Geometry check sheet. Reference: the model listing, model coordinates, mm. Face numbers are marked on the shaded views. Coordinates: 2 decimals unless noted, no trailing zeros. Order: outer loops, then holes, each group sorted by start corner. A loop starts at its lowest first (then second) coordinate and runs counter-clockwise, first axis right, second up.
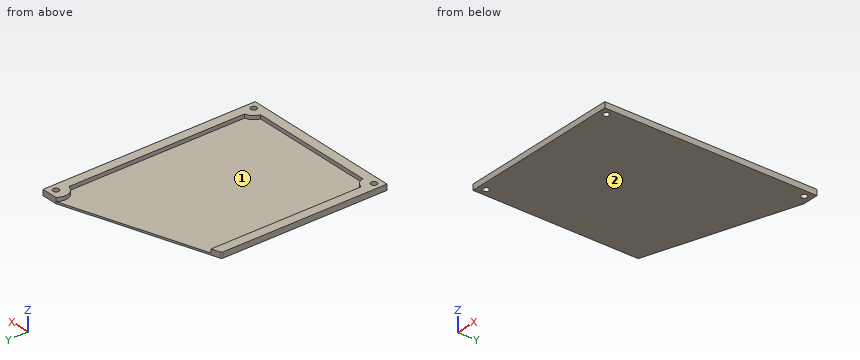
```python
from build123d import *

# Parameters (mm, degrees)
SKETCH_W           = 86.36
SKETCH_H           = 113.03
PAD_DEPTH          = 10
SKETCH001_R        = 1.6
POCKET_DEPTH       = 1
POCKET001_DEPTH    = 9
POCKET002_DEPTH    = 10.001
FILLET_R           = 1
FILLET_FACE20_R    = 1.6
POCKET003_DEPTH    = 9.001
POCKET003_FACE20_R = 1.6
POCKET004_DEPTH    = 9.001
POCKET004_FACE21_R = 1.6
POCKET005_DEPTH    = 9.001
POCKET005_FACE11_R = 1.6
POCKET006_DEPTH    = 7


with BuildPart() as part:
    # Sketch → Pad (new body)
    with BuildSketch(Plane.XY):
        Rectangle(SKETCH_W, SKETCH_H)
    extrude(amount=PAD_DEPTH)

    # Sketch001 (on Face6 of Pad) → Pocket (cut)
    with BuildSketch(Plane.XY.offset(10)):
        with Locations((-39.37, -52.705)):
            Circle(SKETCH001_R)
        with Locations((39.37, -52.705)):
            Circle(SKETCH001_R)
        with Locations((39.37, 52.705)):
            Circle(SKETCH001_R)
    extrude(amount=-POCKET_DEPTH, mode=Mode.SUBTRACT)

    # Sketch002 (on Face5 of Pocket) → Pocket001 (cut)
    with BuildSketch(Plane.XY.offset(10)):
        with BuildLine():
            Line((-38.18, 56.515), (34.734927, 56.515))
            ThreePointArc((34.734927, 56.515), (33.716611, 50.695226), (38.18, 46.824192))
            Line((38.18, -46.824192), (38.18, 46.824192))
            ThreePointArc((38.18, -46.824192), (35.127359, -48.462359), (33.489192, -51.515))
            Line((-33.489192, -51.515), (33.489192, -51.515))
            ThreePointArc((-33.489192, -51.515), (-35.127359, -48.462359), (-38.18, -46.824192))
            Line((-38.18, -46.824192), (-38.18, 56.515))
        make_face()
    extrude(amount=-POCKET001_DEPTH, mode=Mode.SUBTRACT)

    # Sketch003 (on Face2 of Pocket001) → Pocket002 (cut, through all)
    with BuildSketch(Plane(origin=(0, 0, 0), x_dir=(1, 0, 0), z_dir=(0, 0, -1))):
        Polygon((34.734927, -56.515), (-43.18, -31.515), (-75.693622, -36.778853), (-62.654191, -136.900963), (71.529642, -145.781613), align=None)
    extrude(amount=-POCKET002_DEPTH, mode=Mode.SUBTRACT)

    # Fillet
    fillet_edges = [part.edges().sort_by_distance(p)[0] for p in [
        (-43.18, 31.515, 5),
    ]]
    fillet(fillet_edges, radius=FILLET_R)

    # Fillet Face20 → Pocket003 (cut, through all)
    with BuildSketch(Plane(origin=(39.37, 52.705, 9), x_dir=(0, 1, 0), z_dir=(0, 0, 1))):
        Circle(FILLET_FACE20_R)
    extrude(amount=-POCKET003_DEPTH, mode=Mode.SUBTRACT)

    # Pocket003 Face20 → Pocket004 (cut, through all)
    with BuildSketch(Plane(origin=(39.37, -52.705, 9), x_dir=(0, 1, 0), z_dir=(0, 0, 1))):
        Circle(POCKET003_FACE20_R)
    extrude(amount=-POCKET004_DEPTH, mode=Mode.SUBTRACT)

    # Pocket004 Face21 → Pocket005 (cut, through all)
    with BuildSketch(Plane(origin=(-39.37, -52.705, 9), x_dir=(0, 1, 0), z_dir=(0, 0, 1))):
        Circle(POCKET004_FACE21_R)
    extrude(amount=-POCKET005_DEPTH, mode=Mode.SUBTRACT)

    # Pocket005 Face11 → Pocket006 (cut)
    with BuildSketch(Plane(origin=(4.164338, -17.509982, 10), x_dir=(0, 1, 0), z_dir=(0, 0, 1))):
        with BuildLine():
            Line((50.629296, 42.344338), (49.247815, 46.649859))
            ThreePointArc((49.247815, 46.649859), (48.8849, 47.152274), (48.295629, 47.344338))
            Line((48.295629, 47.344338), (-39.005018, 47.344338))
            Line((-39.005018, 47.344338), (-39.005018, -39.015662))
            Line((-39.005018, -39.015662), (74.024982, -39.015662))
            Line((74.024982, -39.015662), (74.024982, -30.570589))
            ThreePointArc((74.024982, -30.570589), (68.205208, -29.552273), (64.334174, -34.015662))
            Line((64.334174, -34.015662), (-29.31421, -34.015662))
            ThreePointArc((-29.31421, -34.015662), (-30.952377, -30.963021), (-34.005018, -29.324854))
            Line((-34.005018, -29.324854), (-34.005018, 37.65353))
            ThreePointArc((-34.005018, 37.65353), (-30.952377, 39.291697), (-29.31421, 42.344338))
            Line((-29.31421, 42.344338), (50.629296, 42.344338))
        make_face()
        with Locations((-35.195018, -35.205662)):
            Circle(POCKET005_FACE11_R, mode=Mode.SUBTRACT)
        with Locations((70.214982, -35.205662)):
            Circle(POCKET005_FACE11_R, mode=Mode.SUBTRACT)
        with Locations((-35.195018, 43.534338)):
            Circle(POCKET005_FACE11_R, mode=Mode.SUBTRACT)
    extrude(amount=-POCKET006_DEPTH, mode=Mode.SUBTRACT)


solid = part.part
```
Item 1: Sectioned sample at C-C (y = -41). Record the cut outline in (x, z).
Item 2: Depth check by flat-ended pin: P1, Ø1.6, axis at x = -4, z = 1.5, coming from the +Y side; P2, Ø1, axis at x = 20.5, y = 9.5, coming from the +Z side; P3, Ø1.5, axis at x = -3, z = 0.5, coming from the +Y side. Enter the tip coordinate at first touch or a pass-through.
Item 3: Sectioned sample at B-B (z = 2.5). Record the cut outline in (x, y) (3 decimals).
Item 4: Release check for a two-part mould opening along X. For the marked faces 1 and 2 record: pulls with the +X half, pulls with the -X half, needs draft (parallel to the pull), parting line crosses it, or undercut.
Item 5: Thickness scan on line 1 along Y through (x, z) = (39.37, 0.8) (3 decimals); line 2 along X through (y, z) = (-25, 1.8); line 3 along Y through (x, z) = (-30, 2.75) (3 decimals). Record the ranges inside material, lowest first.
Item 6: Sectioned sample at A-A (x = 39.37). Record the cut outline in (y, z) (3 decimals), and give its area (3 significant figures).
Item 7: Sectioned sample at D-D (x = -39.37). Record the cut outline in (y, z) (3 decimals).
Geometry check:
1. outline: (-43.18, 0) - (43.18, 0) - (43.18, 3) - (38.18, 3) - (38.18, 1) - (-38.18, 1) - (-38.18, 3) - (-43.18, 3) - close
2. P1: stops at y = 44.29
2. P2: stops at z = 1
2. P3: stops at y = 44.65
3. outline: (-43.18, -56.515) - (43.18, -56.515) - (43.18, 56.515) - (34.735, 56.515) arc R6 ccw to (38.18, 46.824) - (38.18, -46.824) arc R6 ccw to (33.489, -51.515) - (-33.489, -51.515) arc R6 ccw to (-38.18, -46.824) - (-38.18, 33.119) - (-42.486, 31.738) arc R1 ccw to (-43.18, 30.786) - close; hole circle Ø3.2 at (-39.37, -52.705); hole circle Ø3.2 at (39.37, -52.705); hole circle Ø3.2 at (39.37, 52.705)
4. face 1: undercut
4. face 2: needs draft
5. line 1: y = -56.515 to -54.305, -51.105 to 51.105, 54.305 to 56.515
5. line 2: x = -43.18 to -38.18, 38.18 to 43.18
5. line 3: y = -56.515 to -51.515
6. outline: (-56.515, 0) - (-54.305, 0) - (-54.305, 3) - (-56.515, 3) - close; (-51.105, 0) - (51.105, 0) - (51.105, 3) - (-51.105, 3) - close; (54.305, 0) - (56.515, 0) - (56.515, 3) - (54.305, 3) - close
6. area: 320 mm2
7. outline: (-56.515, 0) - (-54.305, 0) - (-54.305, 3) - (-56.515, 3) - close; (-51.105, 0) - (32.737, 0) - (32.737, 3) - (-51.105, 3) - close
